Job drawing, mm, ordinate dimensions from the low corner. One solid piece. A direction names the side the tool comes from. Coordinates: 2 decimals unless noted, no trailing zeros. Order: outer loops, then holes, each group sorted by start corner. A loop starts at its lowest first (then second) coordinate and runs counter-clockwise, first axis right, second up. Notation, with made-up numbers: (38.25, 84.25) - (64.25, 84.25) arc R29 ccw to (64.25, 122.25) - close; hole circle Ø8 at (45, -38). An arc over 180 degrees is marked (long way). Use one line per item in the form item = value.
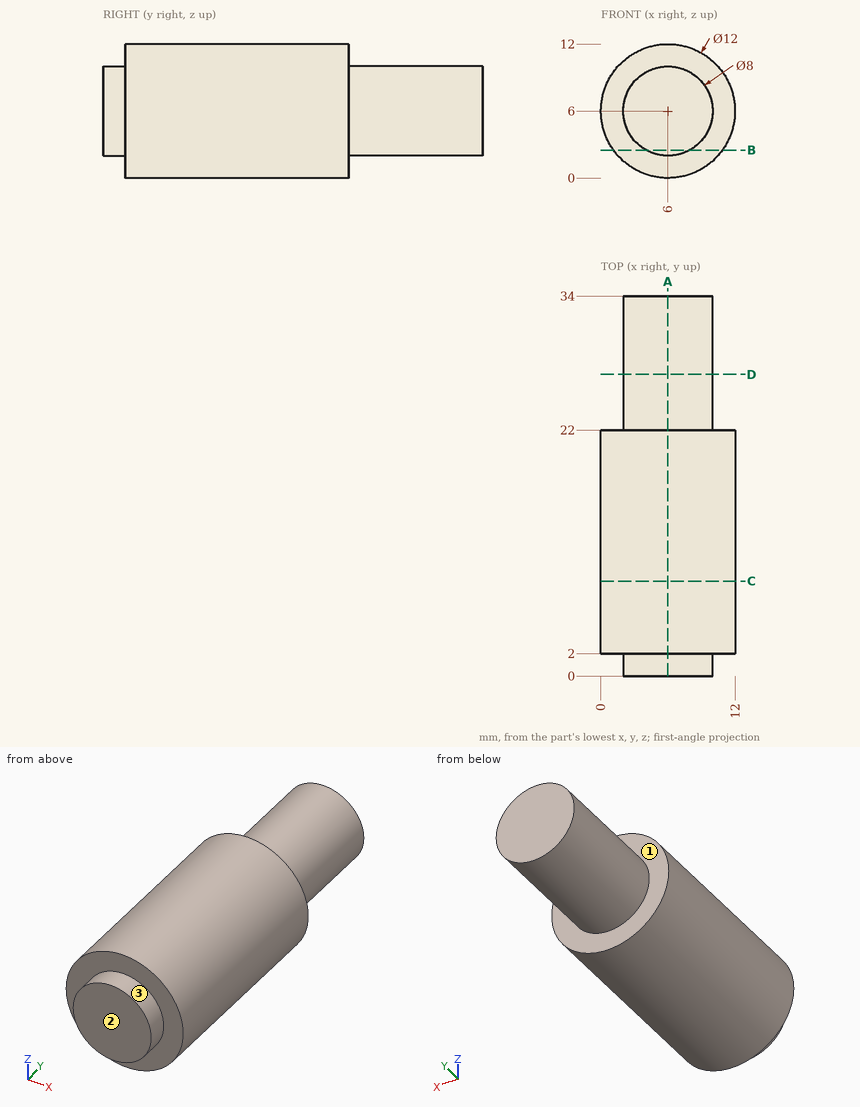
Item 1: Drop flat-ended pins along their axis: pin 1 (3.5 mm diameter, centred on x = 7.5, z = 3.5, fed in from -Y); pin 2 (1 mm diameter, centred on y = 12.5, z = 11, fed in from -X); pin 3 (1 mm diameter, centred on x = 9, y = 25, fed in from +Z); pin 4 (1 mm diameter, centred on y = 7.5, z = 9, fed in from +X). Give the stop position or say it passes through.
Derived:
pin_1 = 0
pin_2 = 2.03
pin_3 = 9.12
pin_4 = 11.45
Item 2: 3-axis set-ups, long thin cutter, end or side, ignore diameter. For the marked faces 1, 2 and 3: which of +Z, -Z, +X, -X, +Y, -Y reach the whole face in a straight line?
Derived:
face_1 = +Y
face_2 = +Z, -Z, +X, -X, -Y
face_3 = -Y
Item 3: Cut at B-B, the plane z = 2.5. Write the cut outline in (x, y), plus the area to 3 significant figures.
Derived:
outline = (1.13, 2) - (4.06, 2) - (4.06, 0) - (7.94, 0) - (7.94, 2) - (10.87, 2) - (10.87, 22) - (7.94, 22) - (7.94, 34) - (4.06, 34) - (4.06, 22) - (1.13, 22) - close
area = 249 mm²
Item 4: Drill centre lines: line 1 (Y direction, x = 1.5, z = 4); line 2 (X direction, y = 12.5, z = 10.25); line 3 (X direction, y = 18.5, z = 7). Where is each one in solid material? Low to high. Write a range as [from, to].
Derived:
line_1 = [2, 22]
line_2 = [1.76, 10.24]
line_3 = [0.08, 11.92]
Item 5: Cut at A-A, the plane x = 6. Write the cut outline in (y, z), plus the area to 3 significant figures.
Derived:
outline = (0, 2) - (2, 2) - (2, 0) - (22, 0) - (22, 2) - (34, 2) - (34, 10) - (22, 10) - (22, 12) - (2, 12) - (2, 10) - (0, 10) - close
area = 352 mm²
Item 6: Cut at C-C, the plane y = 8.5. Write the cut outline in (x, z), plus the area to 3 significant figures.
Derived:
outline = circle Ø12 at (6, 6)
area = 113 mm²
Item 7: Cut at D-D, the plane y = 27. Write the cut outline in (x, z).
Derived:
outline = circle Ø8 at (6, 6)
